Read the model definition and answer for the solid it produces. Units are mm, in the model's axes. A direction names the side the tool comes from. Coordinates: 2 decimals unless noted, no trailing zeros. Order: outer loops, then holes, each group sorted by start corner. A loop starts at its lowest first (then second) coordinate and runs counter-clockwise, first axis right, second up. Notation, with made-up numbers: (79.25, 27) - (91.25, 27) arc R34 cw to (91.25, 58) - close; hole circle Ø11 at (4.5, -17). An arc over 180 degrees is marked (long way). Use one line per item in the form item = value.
```python
from build123d import *

# Parameters (mm, degrees)
SKETCH1_W           = 80
SKETCH1_H           = 20
BOSS_EXTRUDE1_DEPTH = 5
FILLET1_R           = 5
SHELL1_T            = -2
BOSS_EXTRUDE2_DEPTH = 6
SKETCH3_R           = 1.475
CUT_EXTRUDE1_DEPTH  = 4


with BuildPart() as part:
    # Sketch1 → Boss-Extrude1 (new body)
    with BuildSketch(Plane.XY):
        Rectangle(SKETCH1_W, SKETCH1_H)
    extrude(amount=BOSS_EXTRUDE1_DEPTH)

    # Fillet1
    fillet1_edges = [part.edges().sort_by_distance(p)[0] for p in [
        (40, -10, 2.5),
        (-40, -10, 2.5),
        (-40, 10, 2.5),
        (40, 10, 2.5),
    ]]
    fillet(fillet1_edges, radius=FILLET1_R)

    # Shell1
    shell1_openings = [part.faces().sort_by_distance(p)[0] for p in [
        (0, 0, 5),
    ]]
    offset(amount=SHELL1_T, openings=shell1_openings, kind=Kind.INTERSECTION)

    # Sketch2 → Boss-Extrude2 (add)
    with BuildSketch(Plane(origin=(0, 10, 0), x_dir=(1, 0, 0), z_dir=(0, 1, 0))):
        Polygon((0, 0), (-3, 0), (-3, -5), (3, -5), (3, 0), align=None)
    extrude(amount=BOSS_EXTRUDE2_DEPTH)

    # Sketch3 → Cut-Extrude1 (cut)
    with BuildSketch(Plane(origin=(0, 16, 0), x_dir=(1, 0, 0), z_dir=(0, 1, 0))):
        with Locations((0, -2.5)):
            Circle(SKETCH3_R)
    extrude(amount=-CUT_EXTRUDE1_DEPTH, mode=Mode.SUBTRACT)


solid = part.part
```
(1) Straight lines are drawn through the part: L1, parallel to Y at x = 34, z = 2.75; L2, parallel to X at y = 13.55, z = 2.5 (3 decimals); L3, parallel to Z at x = 0, y = 13.75 (3 decimals). For each, find the intervals that lie inside material, in ascending order.
Answer list:
L1 = -10 to -8, 8 to 10
L2 = -3 to -1.475, 1.475 to 3
L3 = 0 to 1.025, 3.975 to 5
(2) Which of the six approach directions +Z, -Z, +X, -X, +Y, -Y give full straight-line access (tool end or side, diameter ignored) to faces 1 (the cylindrical face through (-37.14, -7.1, 3.52)), 2 (the flat face through (19, 10, 2)), 3 (the cylindrical face through (-39, 8, 3)), 4 (the cylindrical face through (38, -9, 3)), 5 (the flat face through (0, 12, 2))?
Answer list:
face_1 = +Z
face_2 = +Z, -Z, +X, +Y
face_3 = +Z, -Z, -X, +Y
face_4 = +Z, -Z, +X, -Y
face_5 = +Y
(3) The mould has two halves that part along Y. Classify faces 6 (the flat face through (40, 0, 2)), 7 (the cylindrical face through (-37.14, 7.1, 3.52)), 8 (the flat face through (0, 16, 0.8)): +Y half, -Y half, draft (parallel to the pull), parting line (faces both ways), or undercut.
Answer list:
face_6 = draft
face_7 = undercut
face_8 = +Y half
(4) Section A-A, the plane x = 0 is taken. Write down the section's boundary in (y, z) (3 decimals), then the cut area to 3 significant figures.
Answer list:
outline = (-10, 0) - (16, 0) - (16, 1.025) - (12, 1.025) - (12, 3.975) - (16, 3.975) - (16, 5) - (8, 5) - (8, 2) - (-8, 2) - (-8, 5) - (-10, 5) - close
area = 70.2 mm2
(5) Section C-C, the plane y = 7 is taken. Write down the section's boundary in (x, z).
Answer list:
outline = (-39.58, 0) - (39.58, 0) - (39.58, 5) - (37.24, 5) - (37.24, 2) - (-37.24, 2) - (-37.24, 5) - (-39.58, 5) - close
(6) Given pin 1 Ø2.5 at (y, z) = (14, 1.5) entering from +X; pin 2 Ø1 at (y, z) = (9.5, 4) entering from -X; pin 3 Ø2.5 at (x, z) = (15.5, 1.5) entering from +Y, each flat-ended and moving along its own axis, determine where each tip first touches the part or whether it passes through.
Answer list:
pin_1 = 3
pin_2 = -38
pin_3 = 10
(7) Section B-B, the plane y = 2.25 is taken. Write down the section's boundary in (x, z), then the cut area to 3 significant figures.
Answer list:
outline = (-40, 0) - (40, 0) - (40, 5) - (38, 5) - (38, 2) - (-38, 2) - (-38, 5) - (-40, 5) - close
area = 172 mm2
